```python
from build123d import *

# Parameters (mm, degrees)
BOSS_EXTRUDE1_DEPTH      = 7.5
BOSS_EXTRUDE1_DEPTH_BACK = 7.5
CUT_EXTRUDE1_DEPTH       = 109.450580006
CUT_EXTRUDE1_DEPTH_BACK  = 109.450580006
SKETCH2_R                = 2.25
SKETCH3_R                = 2.1
SKETCH3_R_2              = 1.6
CUT_EXTRUDE2_DEPTH       = 106.254370403


with BuildPart() as part:
    # Sketch1 → Boss-Extrude1 (new, two sides: drawn at the far end of the back side and taken through both)
    with BuildSketch(Plane(origin=(0, 0, 0), x_dir=(1, 0, 0), z_dir=(0, 1, 0)).offset(-BOSS_EXTRUDE1_DEPTH_BACK)):
        with BuildLine():
            Line((-65.80458146, -35.321832584), (-65.80458146, -81.80458146))
            Line((-65.80458146, -81.80458146), (-50.80458146, -81.80458146))
            Line((-50.80458146, -81.80458146), (-50.80458146, -35.321832584))
            ThreePointArc((-50.80458146, -35.321832584), (-44.852454502, -20.952126958), (-30.482748876, -15))
            Line((-30.482748876, -15), (20, -15))
            Line((20, -15), (20, 0))
            Line((20, 0), (-30.482748876, 0))
            ThreePointArc((-30.482748876, 0), (-55.45905622, -10.34552524), (-65.80458146, -35.321832584))
        make_face()
    extrude(amount=BOSS_EXTRUDE1_DEPTH + BOSS_EXTRUDE1_DEPTH_BACK)

    # Sketch2 → Cut-Extrude1 (cut, two sides: drawn at the far end of the back side and taken through both)
    with BuildSketch(Plane.ZY.offset(50.80458146).offset(-CUT_EXTRUDE1_DEPTH_BACK)):
        with Locations((66.80458146, 0)):
            Circle(SKETCH2_R)
    extrude(amount=CUT_EXTRUDE1_DEPTH + CUT_EXTRUDE1_DEPTH_BACK, mode=Mode.SUBTRACT)

    # Sketch3 → Cut-Extrude2 (cut, through all)
    with BuildSketch(Plane(origin=(0, 0, 0), x_dir=(-1, 0, 0), z_dir=(0, 0, -1))):
        Circle(SKETCH3_R)
        with Locations((-11.5, 0)):
            Circle(SKETCH3_R_2)
        with Locations((11.5, 0)):
            Circle(SKETCH3_R_2)
    extrude(amount=-CUT_EXTRUDE2_DEPTH, mode=Mode.SUBTRACT)

    # Sketch5 → bearing-seats (revolve, cut)
    with BuildSketch(Plane(origin=(0, 0, 0), x_dir=(1, 0, 0), z_dir=(0, 1, 0))):
        with BuildLine():
            Line((-65.80458146, -71.45458146), (-65.20458146, -71.45458146))
            Line((-65.20458146, -71.45458146), (-65.20458146, -70.95458146))
            ThreePointArc((-65.20458146, -70.95458146), (-65.175292138, -70.883870782), (-65.10458146, -70.85458146))
            Line((-65.10458146, -70.85458146), (-62.80458146, -70.85458146))
            Line((-62.80458146, -70.85458146), (-62.80458146, -66.80458146))
            Line((-62.80458146, -66.80458146), (-65.80458146, -66.80458146))
            Line((-65.80458146, -66.80458146), (-65.80458146, -71.45458146))
        make_face()
        with BuildLine():
            Line((-50.80458146, -66.80458146), (-53.80458146, -66.80458146))
            Line((-53.80458146, -66.80458146), (-53.80458146, -70.85458146))
            Line((-53.80458146, -70.85458146), (-51.50458146, -70.85458146))
            ThreePointArc((-51.50458146, -70.85458146), (-51.433870782, -70.883870782), (-51.40458146, -70.95458146))
            Line((-51.40458146, -70.95458146), (-51.40458146, -71.45458146))
            Line((-51.40458146, -71.45458146), (-50.80458146, -71.45458146))
            Line((-50.80458146, -71.45458146), (-50.80458146, -66.80458146))
        make_face()
    revolve(axis=Axis((-84.392341333, 0, 66.80458146), (1, 0, 0)), mode=Mode.SUBTRACT)


solid = part.part
```
Part model, mm, in its own coordinate system. A direction names the side the tool comes from. Round coordinates to 2 decimals unless told otherwise and drop trailing zeros. Write each loop counter-clockwise with the first axis right and the second up, starting at its lowest first coordinate (ties: lowest second). Pieces come first, ordered by that corner, then holes. Notation, with made-up numbers: M -31,87.5 L 16,87.5 A18 cw 16,121.5 Z; hole C -24,41.5 d4. An arc over 180 degrees is marked long. Answer as CSV lines item,"result". Start each with the question number.
1) Drill centre lines: L1, parallel to Z at x = -23, y = 7; L2, parallel to X at y = -3, z = 57.5; L3, parallel to X at y = -3.75, z = 9. Where is each one in solid material? Low to high.
2) Drop flat-ended pins along their axis: pin 1 (1 mm diameter, centred on x = 2.5, y = 5, fed in from +Z); pin 2 (1 mm diameter, centred on x = -34, y = 2, fed in from +Z); pin 3 (4.5 mm diameter, centred on y = 0.5, z = 65.5, fed in from -X); pin 4 (2.5 mm diameter, centred on y = 0, z = 66.8, fed in from +X). Give the stop position or say it passes through.
3) Band-saw the part on C-C (x = 14.5). List the corners of the cut face in (y, z), then the cut area to 3 significant figures.
4) Band-saw the part on B-B (y = 0). Count the separate pieces of the cut face and the enclosed holes in it, then the cut area to 3 significant figures.
5) Band-saw the part on D-D (z = 44). List the corners of the cut face in (x, y).
6) Band-saw the part on A-A (x = -11.5). List the corners of the cut face in (y, z).
7) Which spindle directions (+Z, -Z, +X, -X, +Y, -Y) get a long thin tool onto all of the face, cutting with end or side? Do faces 4 (the face through (-63.94, -0.18, 62.76)), 5 (the face through (-50.805, 0, 59)), 6 (the face through (-52.64, -0.18, 62.76)). Say none if no direction does.
8) Mould opens along Z. For faces 1 (the face through (-51.1, -0.2, 62.16)), 2 (the face through (-6, 0, 15)), 3 (the face through (-55.18, -0.11, 10.07)) say: +Z half, -Z half, draft (parallel to the pull), parting line (faces both ways), or undercut.
Worked out:
1,L1,"0 to 15"
1,L2,"-65.8 to -50.8"
1,L3,"-54.04 to 20"
2,pin 1,"z = 15"
2,pin 2,"z = 15.4"
2,pin 3,"x = -62.8"
2,pin 4,"through"
3,outline,"M -7.5,0 L 7.5,0 L 7.5,15 L -7.5,15 Z"
3,area,"225 mm²"
4,separate pieces,"5"
4,enclosed holes,"0"
4,area,"1,860 mm²"
5,outline,"M -65.8,-7.5 L -50.8,-7.5 L -50.8,7.5 L -65.8,7.5 Z"
6,outline,"M -7.5,0 L -1.6,0 L -1.6,15 L -7.5,15 Z; M 1.6,0 L 7.5,0 L 7.5,15 L 1.6,15 Z"
7,face 4,"-X"
7,face 5,"+Z, +X, +Y, -Y"
7,face 6,"+X"
8,face 1,"undercut"
8,face 2,"+Z half"
8,face 3,"-Z half"
